Source: three-view drawing plus pictorial views. Frame: mm from the lowest corner of the part. A direction names the side the tool comes from. Give positions to 0.01 mm unless a question says otherwise; leave off trailing zeros. Loops run counter-clockwise (first coordinate to the right, second up) from the corner with the lowest first, then second, coordinate; pieces in that order, holes last. Notation, with made-up numbers: (48, 35) - (61, 35) arc R15 ccw to (61, 63) - close; hole circle Ø7 at (-23, 35.5). An arc over 180 degrees is marked (long way). One line per item, written item: value.
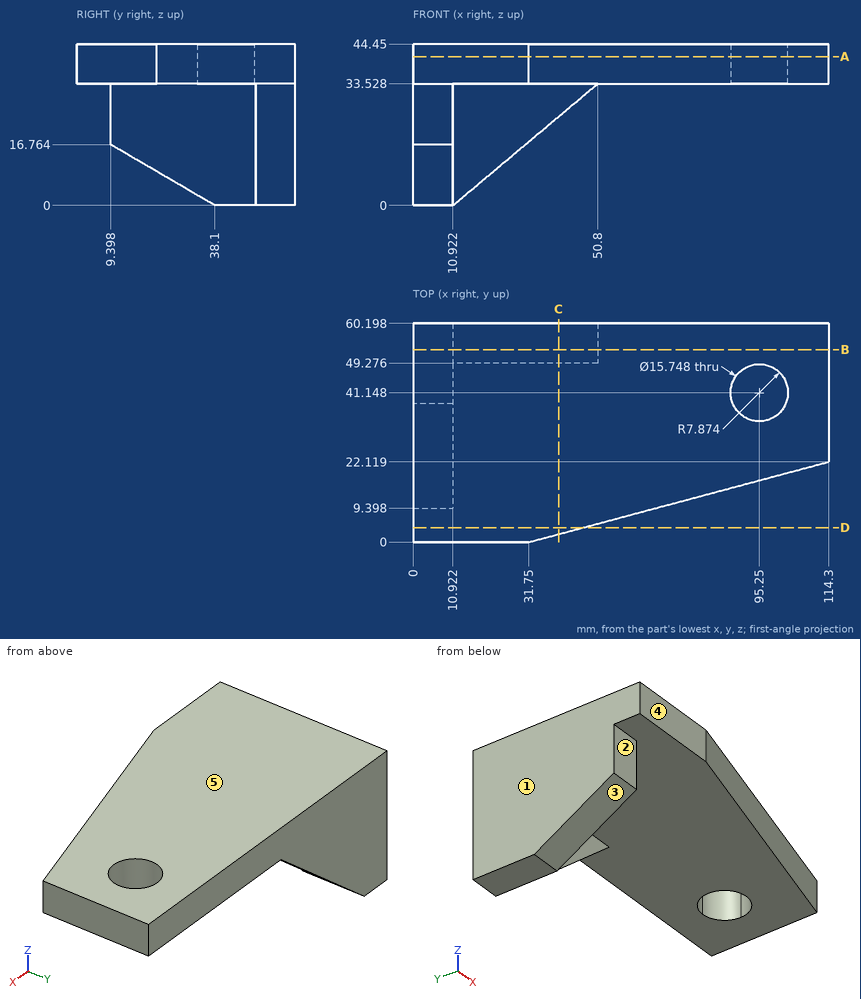
Item 1: Access query for the marked faces 1 and 2. Directions: +Z, -Z, +X, -X, +Y, -Y. A direction counts if a zero-diameter tool reaches every point of the face in a straight line with its end or side. Return the directions, or none.
Verdict:
face 1: +Z, -Z, -X, +Y, -Y
face 2: -Z, +X, -X, -Y
Item 2: Material intervals for L1, parallel to Z at x = 40, y = 48; L2, parallel to X at y = 48, z = 3; L3, parallel to Y at x = 15, z = 8, sorted ascending.
Verdict:
L1: z = 33.53 to 44.45
L2: x = 0 to 10.92
L3: y = 49.28 to 60.2
Item 3: Draft query along Z for the marked faces 3, 4 and 5. Return one class per face: pulls with the +Z half, pulls with the -Z half, needs draft (parallel to the pull), parting line crosses it, or undercut.
Verdict:
face 3: pulls with the -Z half
face 4: needs draft
face 5: pulls with the +Z half
Item 4: Section A-A, the plane z = 41. Output: boundary loops of the cut face in (x, y), and give its area (3 significant figures).
Verdict:
outline: (0, 0) - (31.75, 0) - (114.3, 22.12) - (114.3, 60.2) - (0, 60.2) - close; hole circle Ø15.75 at (95.25, 41.15)
area: 5,770 mm^2
Item 5: Section B-B, the plane y = 53. Output: boundary loops of the cut face in (x, z), and give its area (3 significant figures).
Verdict:
outline: (0, 0) - (10.92, 0) - (50.8, 33.53) - (114.3, 33.53) - (114.3, 44.45) - (0, 44.45) - close
area: 2,280 mm^2
Item 6: Section C-C, the plane x = 40. Output: boundary loops of the cut face in (y, z).
Verdict:
outline: (2.21, 33.53) - (49.28, 33.53) - (49.28, 24.45) - (60.2, 24.45) - (60.2, 44.45) - (2.21, 44.45) - close
Item 7: Pin query (flat end, axial travel): P1, Ø12, axis at y = 8.5, z = 19, coming from the -X side; P2, Ø8.5, axis at x = 7.5, z = 26.5, coming from the -Y side; P3, Ø18, axis at x = 71.5, y = 20.5, coming from the -Z side; P4, Ø10, axis at x = 50, z = 24, coming from the -Y side. Return the tip coordinate at first contact, or that it passes through.
Verdict:
P1: stops at x = 0
P2: stops at y = 9.4
P3: stops at z = 33.53
P4: passes through
Item 8: Section D-D, the plane y = 4. Output: boundary loops of the cut face in (x, z), and give its area (3 significant figures).
Verdict:
outline: (0, 33.53) - (46.68, 33.53) - (46.68, 44.45) - (0, 44.45) - close
area: 510 mm^2
